Autodesk Inventor part; units mm, degrees
ref_plane "YZ Plane" through (0, 0, 0) normal (1, 0, 0) x (0, 1, 0)
ref_plane "XZ Plane" through (0, 0, 0) normal (0, 1, 0) x (-1, 0, 0)
ref_plane "XY Plane" through (0, 0, 0) normal (0, 0, 1) x (1, 0, 0)
sketch "草图1" plane through (0, 0, 0) normal (0, 1, 0) x (-1, 0, 0)
  line L0 (0, 0) -> (13, 0)
  line L1 (13, 0) -> (13, 3)
  line L2 (13, 3) -> (7, 3)
  line L3 (7, 3) -> (7, 4.5)
  line L4 (7, 4.5) -> (8, 4.5)
  line L5 (8, 4.5) -> (8, 15)
  line L6 (8, 15) -> (0, 15)
  line L7 (0, 15) -> (0, 0)
  dimension "d0" = 13
  dimension "d2" = 3
  dimension "d3" = 1.5
  dimension "d4" = 1
  dimension "d5" = 8
  dimension "d6" = 12
revolve "旋转1" add sketch "草图1" angle 360 about axis through (0, 0, 15) along (0, 0, -1)
chamfer "倒角1" distance 1 angle 45 1 edges at (8, 0, 15)
thread "螺纹1"
sketch "草图2" plane through (0, 0, 0) normal (0, 0, -1) x (-1, 0, 0)
  circle A0 centre (0, 0) radius 8
  line L0 (9.815, 0) -> (4.9075, -8.5)
  line L1 (4.9075, -8.5) -> (-4.9075, -8.5)
  line L2 (-4.9075, -8.5) -> (-9.815, 0)
  line L3 (-9.815, 0) -> (-4.9075, 8.5)
  line L4 (-4.9075, 8.5) -> (4.9075, 8.5)
  line L5 (4.9075, 8.5) -> (9.815, 0)
  point P0 (0, 0)
  dimension "d13" = 17
extrude "拉伸1" add sketch "草图2" along normal blind 10 contours A0 | L0 L1 L2 L3 L4 L5
fillet "圆角1" radius 1.5 6 edges at (0, -8.5, -10) (7.3612, -4.25, -10) (7.3612, 4.25, -10) (0, 8.5, -10) (-7.3612, 4.25, -10) (-7.3612, -4.25, -10)
equation "\"d0\" = 0.5 * D0"
equation "\"d2\" = a"
equation "\"d5\" = 0.5 * d"
equation "\"d6\" = l_"
equation "\"d\" = 16"
equation "\"D0\" = 26"
equation "\"L\" = 23"
equation "\"l_\" = 12"
equation "\"a\" = 3"
equation "\"D\" = 19.6"
equation "\"S_\" = 17"
equation "\"D1\" = 16.2"
equation "\"d1\" = 17"
equation "\"H_\" = 2"
properties part number "排油孔螺塞" material "钢，软"
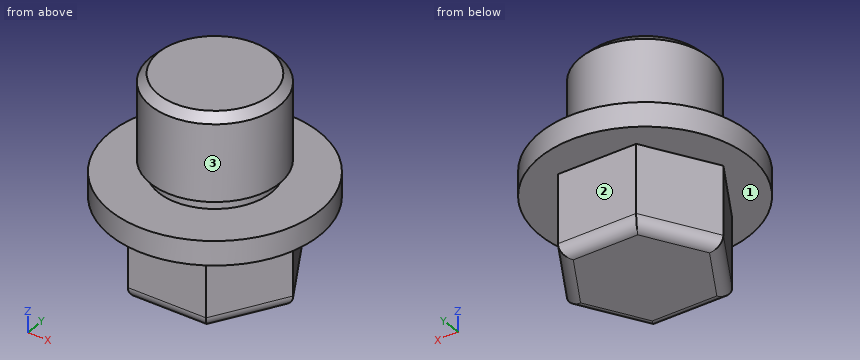
Geometry: final body of the model. Coordinates: model frame, mm. Face numbers are marked on the shaded views. A direction names the side the tool comes from. Round coordinates to 2 decimals unless told otherwise and drop trailing zeros. Loops run counter-clockwise (first coordinate to the right, second up) from the corner with the lowest first, then second, coordinate; pieces in that order, holes last. Notation, with made-up numbers: (30, 75) -> (78, 75) arc R19 ccw to (78, 102) -> close; hole circle Ø6 at (-12.5, 78.5). An arc over 180 degrees is marked (long way). Use one line per item in the form item = value. Start each with the question number.
1) First-contact query: P1, Ø8, axis at x = 0.5, z = -7.5, coming from the -Y side; P2, Ø9.5, axis at x = 1.5, z = -5.5, coming from the +Y side; P3, Ø1, axis at x = -7.5, z = 2, coming from the -Y side; P4, Ø6, axis at x = -8.5, y = 0.5, coming from the -Z side. Flat tips, straight axial feed; report the tip coordinate or a pass-through.
2) Access query for the marked faces 1, 2 and 3. Directions: +Z, -Z, +X, -X, +Y, -Y. A direction counts if a zero-diameter tool reaches every point of the face in a straight line with its end or side. Return the directions, or none.
3) Section C-C on z = 1. Output: boundary loops of the cut face in (x, y), then the cut area to 3 significant figures.
4) Section B-B on z = -8. Output: boundary loops of the cut face in (x, y) (1 decimal), then the cut area to 3 significant figures.
5) Section D-D on y = 9.5. Output: boundary loops of the cut face in (x, z), then the cut area to 3 significant figures.
6) Line query: L1, parallel to Z at x = 6.25, y = 8.75; L2, parallel to Z at x = 4.5, y = -6; L3, parallel to Y at x = -1, z = 13.25. Output: solid intervals per line, ascending.
7) Section A-A on x = 0. Output: boundary loops of the cut face in (y, z).
Response:
q1.P1 = -8.5
q1.P2 = 8.5
q1.P3 = -10.95
q1.P4 = -10
q2.face_1 = -Z
q2.face_2 = -Z, +X, -X, +Y
q2.face_3 = +Z
q3.outline = circle Ø26 at (0, 0)
q3.area = 531 mm^2
q4.outline = (-9.8, 0) -> (-4.9, -8.5) -> (4.9, -8.5) -> (9.8, 0) -> (4.9, 8.5) -> (-4.9, 8.5) -> close
q4.area = 250 mm^2
q5.outline = (-8.87, 0) -> (8.87, 0) -> (8.87, 3) -> (-8.87, 3) -> close
q5.area = 53.2 mm^2
q6.L1 = 0 to 3
q6.L2 = -10 to 3, 4.5 to 14.5
q6.L3 = -7.94 to 7.94
q7.outline = (-13, 0) -> (-8.5, 0) -> (-8.5, -8.5) arc R1.5 ccw to (-7, -10) -> (7, -10) arc R1.5 ccw to (8.5, -8.5) -> (8.5, 0) -> (13, 0) -> (13, 3) -> (7, 3) -> (7, 4.5) -> (8, 4.5) -> (8, 14) -> (7, 15) -> (-7, 15) -> (-8, 14) -> (-8, 4.5) -> (-7, 4.5) -> (-7, 3) -> (-13, 3) -> close
